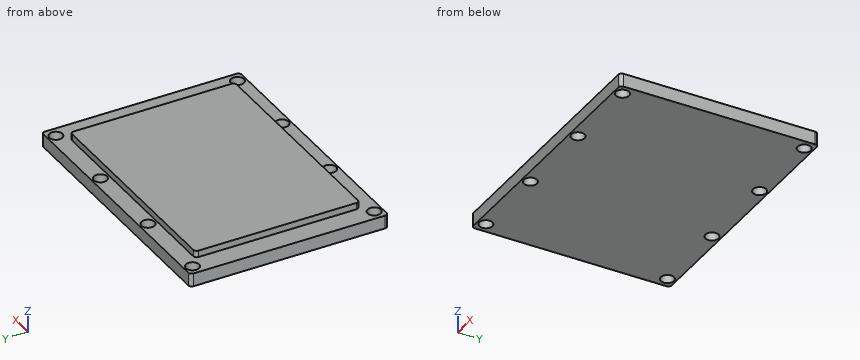
```python
from build123d import *

# Parameters (mm, degrees)
SKETCH_W     = 40
SKETCH_H     = 30
PAD_DEPTH    = 2
SKETCH001_W  = 33.6
SKETCH001_H  = 24.9
PAD001_DEPTH = 1
SKETCH002_R  = 1
POCKET_DEPTH = 2
FILLET_R     = 0.5


with BuildPart() as part:
    # Sketch → Pad (new body)
    with BuildSketch(Plane.XY.offset(2)):
        Rectangle(SKETCH_W, SKETCH_H)
    extrude(amount=PAD_DEPTH)

    # Sketch001 (on Face6 of Pad) → Pad001 (join)
    with BuildSketch(Plane.XY.offset(4)):
        Rectangle(SKETCH001_W, SKETCH001_H)
    extrude(amount=PAD001_DEPTH)

    # Sketch002 → Pocket (cut)
    with BuildSketch(Plane.XY.offset(2)):
        with Locations((-18.4, 13.75)):
            Circle(SKETCH002_R)
        with Locations((-6.4, 13.75)):
            Circle(SKETCH002_R)
        with Locations((6.4, 13.75)):
            Circle(SKETCH002_R)
        with Locations((18.4, 13.75)):
            Circle(SKETCH002_R)
        with Locations((18.4, -13.75)):
            Circle(SKETCH002_R)
        with Locations((6.4, -13.75)):
            Circle(SKETCH002_R)
        with Locations((-6.4, -13.75)):
            Circle(SKETCH002_R)
        with Locations((-18.4, -13.75)):
            Circle(SKETCH002_R)
    extrude(amount=POCKET_DEPTH, mode=Mode.SUBTRACT)

    # Fillet
    fillet_edges = [part.edges().sort_by_distance(p)[0] for p in [
        (20, 15, 3),
        (16.8, 12.45, 4.5),
        (20, -15, 3),
        (16.8, -12.45, 4.5),
        (-20, -15, 3),
        (-16.8, -12.45, 4.5),
        (-20, 15, 3),
        (-16.8, 12.45, 4.5),
    ]]
    fillet(fillet_edges, radius=FILLET_R)


solid = part.part
```
Check sheet for the modelled part. Datum: model origin and axes. Units: mm. Coordinates: 2 decimals unless noted, no trailing zeros. Loops run counter-clockwise (first coordinate to the right, second up) from the corner with the lowest first, then second, coordinate; pieces in that order, holes last.
1) Sectioned sample at D-D (y = 0.5). Record the boundary of the cut face in (x, z), and give its area (3 significant figures).
2) Sectioned sample at B-B (y = -13.75). Record the boundary of the cut face in (x, z).
3) Sectioned sample at A-A (x = 6.4). Record the boundary of the cut face in (y, z), and give its area (3 significant figures).
4) Material ranges on probe 1 along Y at (x, z) = (6.4, 2.55); probe 2 along Y at (x, z) = (6, 4.4); probe 3 along X at (y, z) = (9.5, 4.55), recorded low to high.
5) Gauge pin test, flat ends, axial feed: pin 1 (0.8 mm diameter, centred on x = 0.5, z = 4.5, fed in from +Y); pin 2 (0.5 mm diameter, centred on y = 1, z = 4.5, fed in from -X); pin 3 (2.5 mm diameter, centred on x = -18.4, y = 13.75, fed in from +Z). Record the tip position at first contact, or that the pin passes through.
6) Sectioned sample at C-C (z = 3.25). Count the separate pieces of the cut face and the enclosed holes in it, and give its area (3 significant figures).
Check sheet entries:
1. outline: (-20, 2) - (20, 2) - (20, 4) - (16.8, 4) - (16.8, 5) - (-16.8, 5) - (-16.8, 4) - (-20, 4) - close
1. area: 114 mm2
2. outline: (-20, 2) - (-19.4, 2) - (-19.4, 4) - (-20, 4) - close; (-17.4, 2) - (-7.4, 2) - (-7.4, 4) - (-17.4, 4) - close; (-5.4, 2) - (5.4, 2) - (5.4, 4) - (-5.4, 4) - close; (7.4, 2) - (17.4, 2) - (17.4, 4) - (7.4, 4) - close; (19.4, 2) - (20, 2) - (20, 4) - (19.4, 4) - close
3. outline: (-15, 2) - (-14.75, 2) - (-14.75, 4) - (-15, 4) - close; (-12.75, 2) - (12.75, 2) - (12.75, 4) - (12.45, 4) - (12.45, 5) - (-12.45, 5) - (-12.45, 4) - (-12.75, 4) - close; (14.75, 2) - (15, 2) - (15, 4) - (14.75, 4) - close
3. area: 76.9 mm2
4. probe 1: y = -15 to -14.75, -12.75 to 12.75, 14.75 to 15
4. probe 2: y = -12.45 to 12.45
4. probe 3: x = -16.8 to 16.8
5. pin 1: stops at y = 12.45
5. pin 2: stops at x = -16.8
5. pin 3: stops at z = 4
6. separate pieces: 1
6. enclosed holes: 8
6. area: 1,170 mm2
